Source: CAD feature listing. Evaluate the final solid. Frame: model axes, mm. Round coordinates to 2 decimals unless told otherwise and drop trailing zeros. Write each loop counter-clockwise with the first axis right and the second up, starting at its lowest first coordinate (ties: lowest second). Pieces come first, ordered by that corner, then holes. Notation, with made-up numbers: M 27,34.25 L 45,34.25 A12 cw 45,47.25 Z; hole C 40.25,-14.75 d11. An arc over 180 degrees is marked long. Use a Markdown table: item, result.
```python
from build123d import *

# Parameters (mm, degrees)
SKETCH_1_R          = 1.6
SKETCH_1_R_2        = 1.35
EXTRUDE_1_DEPTH     = 2
CUT_EXTRUDE_1_REACH = 62.829
SKETCH_2_W          = 38
SKETCH_2_H          = 12.009324428


with BuildPart() as part:
    # 草图1 → 凸台-拉伸1 (new body)
    with BuildSketch(Plane(origin=(0, 0, 0), x_dir=(1, 0, 0), z_dir=(0, 1, 0))):
        Polygon((-40.4, -27), (40.4, -27), (50.4, -27), (50.4, 27), (50.4, 34), (-50.4, 34), (-50.4, 27), (-50.4, -27), align=None)
        with Locations(Location((-48, 31.5, 0), (0, 0, 270))):
            Circle(SKETCH_1_R, mode=Mode.SUBTRACT)
        with Locations(Location((-37.6, 24.5, 0), (0, 0, 270))):
            Circle(SKETCH_1_R_2, mode=Mode.SUBTRACT)
        with Locations(Location((-43.9, -24.8, 0), (0, 0, 270))):
            Circle(SKETCH_1_R_2, mode=Mode.SUBTRACT)
        with Locations(Location((37.6, 24.5, 0), (0, 0, 90))):
            Circle(SKETCH_1_R_2, mode=Mode.SUBTRACT)
        with Locations(Location((43.9, -24.8, 0), (0, 0, 90))):
            Circle(SKETCH_1_R_2, mode=Mode.SUBTRACT)
        with Locations(Location((-48, -8.5, 0), (0, 0, 270))):
            Circle(SKETCH_1_R, mode=Mode.SUBTRACT)
        with Locations(Location((48, -8.5, 0), (0, 0, 90))):
            Circle(SKETCH_1_R, mode=Mode.SUBTRACT)
        with Locations(Location((48, 31.5, 0), (0, 0, 90))):
            Circle(SKETCH_1_R, mode=Mode.SUBTRACT)
        with Locations(Location((-37.6, 2.5, 0), (0, 0, 270))):
            Circle(SKETCH_1_R_2, mode=Mode.SUBTRACT)
        with Locations(Location((37.6, 2.5, 0), (0, 0, 90))):
            Circle(SKETCH_1_R_2, mode=Mode.SUBTRACT)
        with BuildLine():
            Line((-21, 22), (21, 22))
            ThreePointArc((21, 22), (25, 18), (21, 14))
            Line((21, 14), (-21, 14))
            ThreePointArc((-21, 14), (-25, 18), (-21, 22))
        make_face(mode=Mode.SUBTRACT)
        with BuildLine():
            Line((-21, 4), (21, 4))
            ThreePointArc((21, 4), (25, 0), (21, -4))
            Line((21, -4), (-21, -4))
            ThreePointArc((-21, -4), (-25, 0), (-21, 4))
        make_face(mode=Mode.SUBTRACT)
    extrude(amount=EXTRUDE_1_DEPTH)

    # 草图2 → 切除-拉伸1 (cut, up to next)
    with BuildSketch(Plane.XZ, mode=Mode.PRIVATE) as cut_extrude_1_sk1:
        with Locations((19, 28.004662214)):
            Rectangle(SKETCH_2_W, SKETCH_2_H)
    cut_extrude_1_tool1 = extrude(cut_extrude_1_sk1.sketch, amount=-CUT_EXTRUDE_1_REACH, mode=Mode.PRIVATE) & part.part
    add(cut_extrude_1_tool1.solids().sort_by_distance((19, 0, 28.004662))[0], mode=Mode.SUBTRACT)


solid = part.part
```
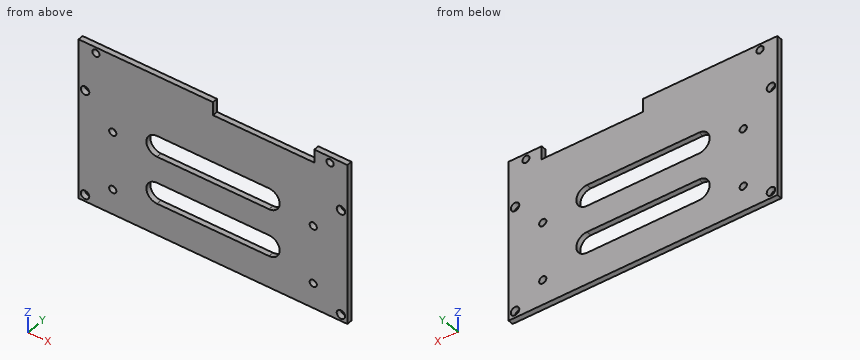
Q1. Line query: L1, parallel to X at y = 0.55, z = -31.5; L2, parallel to X at y = 1.15, z = 24.8; L3, parallel to Z at x = -19, y = 1.9. Output: solid intervals per line, ascending.
Results are:
| item | result |
|---|---|
| L1 | -50.4 to -49.6, -46.4 to 46.4, 49.6 to 50.4 |
| L2 | -50.4 to -45.25, -42.55 to 0, 38 to 42.55, 45.25 to 50.4 |
| L3 | -34 to -22, -14 to -4, 4 to 27 |
Q2. Section B-B on z = -24.5. Return loops of the section in (x, y), plus the area to 3 significant figures.
Results are:
| item | result |
|---|---|
| outline | M -50.4,0 L -38.95,0 L -38.95,2 L -50.4,2 Z; M -36.25,0 L 36.25,0 L 36.25,2 L -36.25,2 Z; M 38.95,0 L 50.4,0 L 50.4,2 L 38.95,2 Z |
| area | 191 mm^2 |
Q3. Section A-A on x = 5. Return loops of the section in (y, z), plus the area to 3 significant figures.
Results are:
| item | result |
|---|---|
| outline | M 0,-34 L 2,-34 L 2,-22 L 0,-22 Z; M 0,-14 L 2,-14 L 2,-4 L 0,-4 Z; M 0,4 L 2,4 L 2,22 L 0,22 Z |
| area | 80.0 mm^2 |
Q4. Section C-C on x = 43.9. Return loops of the section in (y, z).
Results are:
| item | result |
|---|---|
| outline | M 0,-34 L 2,-34 L 2,23.45 L 0,23.45 Z; M 0,26.15 L 2,26.15 L 2,27 L 0,27 Z |
Q5. Section D-D on z = -18. Return loops of the section in (x, y).
Results are:
| item | result |
|---|---|
| outline | M -50.4,0 L -25,0 L -25,2 L -50.4,2 Z; M 25,0 L 50.4,0 L 50.4,2 L 25,2 Z |
Q6. First-contact query: pin 1 Ø3 at (x, z) = (24.5, 0) entering from -Y; pin 2 Ø1 at (x, y) = (2.5, 1) entering from +Z. Flat tips, straight axial feed; report the tip coordinate or a pass-through.
Results are:
| item | result |
|---|---|
| pin 1 | y = 0 |
| pin 2 | z = 22 |
